from build123d import *

# Parameters (mm, degrees)
BOSS_EXTRUDE6_DEPTH = 5.08
FILLET21_R          = 2.54
FILLET22_R          = 2.54
FILLET23_R          = 2.54
FILLET24_R          = 2.54


with BuildPart() as part:
    # Sketch1 → Boss-Extrude6 (new body)
    with BuildSketch(Plane.XY):
        with BuildLine():
            Line((0.14834484, -16.543006694), (-0.005888561, -3.843943262))
            add(Edge.make_bspline(
                [(6.500180425, 78.706993306), (18.901808207, 35.989935529), (-0.005888561, -3.843943262)],
                knots=[0, 0, 0, 1, 1, 1], degree=2))
            Line((6.500180425, 78.706993306), (6.500180425, 85.056993306))
            Line((6.500180425, 85.056993306), (18.406430425, 85.056993306))
            Line((18.406430425, 85.056993306), (22.903074533, 81.262968128))
            Line((22.903074533, 81.262968128), (22.903074533, 55.862968128))
            Line((22.903074533, 55.862968128), (27.983074533, 55.862968128))
            Line((27.983074533, 55.862968128), (27.983074533, 81.262968128))
            Line((27.983074533, 81.262968128), (32.479718641, 85.056993306))
            Line((32.479718641, 85.056993306), (55.223636327, 85.056993306))
            Line((55.223636327, 85.056993306), (55.223636327, 81.262968128))
            add(Edge.make_bspline(
                [(55.223636327, 81.262968128), (27.243001732, 39.093980891), (50.892037627, -3.843943262)],
                knots=[0, 0, 0, 1, 1, 1], degree=2))
            Line((50.892037627, -3.843943262), (50.737804225, -16.543006694))
            Line((50.737804225, -16.543006694), (48.197804225, -16.543006694))
            Line((48.197804225, -16.543006694), (48.197804225, -21.623006694))
            Line((48.197804225, -21.623006694), (43.117804225, -21.623006694))
            Line((43.117804225, -21.623006694), (43.117804225, -16.543006694))
            Line((43.117804225, -16.543006694), (40.577804225, -16.543006694))
            add(Edge.make_bspline(
                [(27.983074533, 5.062968128), (40.683819064, -1.22119794), (40.577804225, -16.543006694)],
                knots=[0, 0, 0, 1, 1, 1], degree=2))
            Line((27.983074533, 5.062968128), (22.903074533, 5.062968128))
            add(Edge.make_bspline(
                [(22.903074533, 5.062968128), (10.202330001, -1.22119794), (10.30834484, -16.543006694)],
                knots=[0, 0, 0, 1, 1, 1], degree=2))
            Line((10.30834484, -16.543006694), (7.76834484, -16.543006694))
            Line((7.76834484, -16.543006694), (7.76834484, -21.623006694))
            Line((7.76834484, -21.623006694), (2.68834484, -21.623006694))
            Line((2.68834484, -21.623006694), (2.68834484, -16.543006694))
            Line((2.68834484, -16.543006694), (0.14834484, -16.543006694))
        make_face()
    extrude(amount=BOSS_EXTRUDE6_DEPTH)

    # Fillet21
    fillet21_edges = [part.edges().sort_by_distance(p)[0] for p in [
        (22.903074533, 81.262968128, 2.54),
    ]]
    fillet(fillet21_edges, radius=FILLET21_R)

    # Fillet22
    fillet22_edges = [part.edges().sort_by_distance(p)[0] for p in [
        (27.983074533, 81.262968128, 2.54),
    ]]
    fillet(fillet22_edges, radius=FILLET22_R)

    # Fillet23
    fillet23_edges = [part.edges().sort_by_distance(p)[0] for p in [
        (6.500180425, 85.056993306, 2.54),
    ]]
    fillet(fillet23_edges, radius=FILLET23_R)

    # Fillet24
    fillet24_edges = [part.edges().sort_by_distance(p)[0] for p in [
        (55.223636327, 85.056993306, 2.54),
    ]]
    fillet(fillet24_edges, radius=FILLET24_R)


solid = part.part
The listing builds one solid part. Answer for the finished solid, in the listing's coordinates (mm). A direction names the side the tool comes from. Give positions to 0.01 mm unless a question says otherwise; leave off trailing zeros. One line per question, with ' | ' between items. Start each with the question number.
1. Straight lines are drawn through the part: line 1 (Y direction, x = 48.5, z = 1.5); line 2 (X direction, y = -5.5, z = 0.75); line 3 (Y direction, x = 23, z = 2.65). For each, find the intervals that lie inside material, in ascending order.
2. Determine the mould class of faces 1 (the face through (48.198, -19, 3)), 2 (the face through (6.5, 81, 3)), 3 (the face through (43.118, -19, 3)), 4 (the face through (28, 44, 5.08)) for opening direction X: +X half, -X half, draft (parallel to the pull), parting line (faces both ways), or undercut.
3. Given P1, Ø3, axis at y = 61.5, z = 2, coming from the +X side; P2, Ø0.8, axis at x = 1, z = 2, coming from the -Y side; P3, Ø3, axis at x = 36, z = 3, coming from the -Y side, each flat-ended and moving along its own axis, determine where each tip first touches the part or whether it passes through.
4. For faces 5 (the face through (2.688, -19, 3)), 6 (the face through (25, 5.063, 3)), 7 (the face through (25, 55.863, 3)), 8 (the face through (49, -16.543, 3)), determine the directions among +Z, -Z, +X, -X, +Y, -Y from which every point of the face is accessible in a straight line to the end or side of a thin tool.
Result:
1) line 1: y = -16.54 to 0.77, 69.64 to 85.06 | line 2: x = 0.01 to 12.37, 38.51 to 50.87 | line 3: y = 5.06 to 55.86
2) face 1: +X half | face 2: -X half | face 3: undercut | face 4: draft
3) P1: stops at x = 45.54 | P2: stops at y = -16.54 | P3: stops at y = -3.51
4) face 5: +Z, -Z, -X, -Y | face 6: +Z, -Z, -Y | face 7: +Z, -Z, +Y | face 8: +Z, -Z, +X, -Y
